Build history of the part. All positions in model axes, mm. Face numbers are marked on the shaded views. A direction names the side the tool comes from. Round coordinates to 2 decimals unless told otherwise and drop trailing zeros. Write each loop counter-clockwise with the first axis right and the second up, starting at its lowest first coordinate (ties: lowest second). Pieces come first, ordered by that corner, then holes. Notation, with made-up numbers: (-16.5, 31) -> (4.5, 31) arc R21 cw to (4.5, 37) -> close; hole circle Ø3 at (39.25, -28.75). An arc over 180 degrees is marked (long way). Answer as CSV lines item,"result".
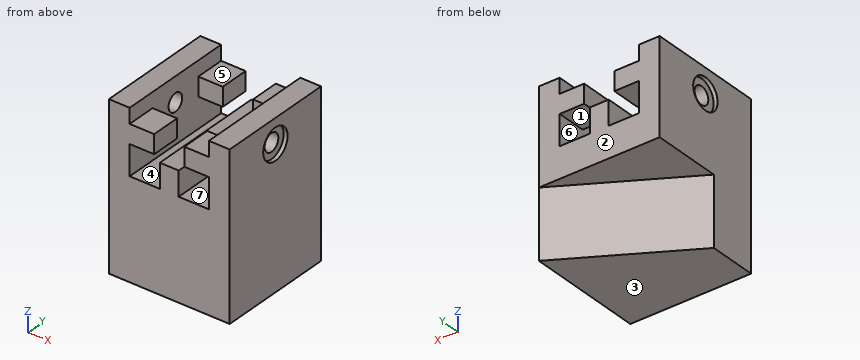
from build123d import *

# Parameters (mm, degrees)
BOSS_EXTRU_1_DEPTH                                = 15
ESQUISSE2_W                                       = 30.8
ESQUISSE2_H                                       = 30
BOSS_EXTRU_2_DEPTH                                = 20
ENL_V_MAT_EXTRU_2_DEPTH                           = 47.870913155
ENL_V_MAT_EXTRU_2_DEPTH_BACK                      = 17.5
ESQUISSE4_W                                       = 4.8
ESQUISSE4_H                                       = 15
ENL_V_MAT_EXTRU_3_DEPTH                           = 6.25
ESQUISSE5_W                                       = 4.8
ESQUISSE5_H                                       = 15
ENL_V_MAT_EXTRU_4_DEPTH                           = 6.25
CHAMBRAGE_POUR_VIS_SIX_PANS_CREUX_M41_D           = 4.5
CHAMBRAGE_POUR_VIS_SIX_PANS_CREUX_M41_DEPTH       = 5.3
CHAMBRAGE_POUR_VIS_SIX_PANS_CREUX_M41_CBORE_D     = 8
CHAMBRAGE_POUR_VIS_SIX_PANS_CREUX_M41_CBORE_DEPTH = 1
CHAMBRAGE_POUR_VIS_SIX_PANS_CREUX_M43_D           = 4.5
CHAMBRAGE_POUR_VIS_SIX_PANS_CREUX_M43_CBORE_D     = 8
CHAMBRAGE_POUR_VIS_SIX_PANS_CREUX_M43_CBORE_DEPTH = 1


with BuildPart() as part:
    # Base → Boss.-Extru.1 (new, symmetric)
    with BuildSketch(Plane(origin=(0, 0, 0), x_dir=(1, 0, 0), z_dir=(0, 1, 0))):
        Polygon((-3.85, -2.4), (-3.85, 2.4), (-10.1, 2.4), (-10.1, 10.1), (-2.4, 10.1), (-2.4, 3.85), (2.4, 3.85), (2.4, 10.1), (10.1, 10.1), (10.1, 2.4), (3.85, 2.4), (3.85, -2.4), (10.1, -2.4), (10.1, -6.25), (15.4, -6.25), (15.4, 15.4), (-15.4, 15.4), (-15.4, -6.25), (-10.1, -6.25), (-10.1, -2.4), align=None)
    extrude(amount=BOSS_EXTRU_1_DEPTH, both=True)

    # Esquisse2 → Boss.-Extru.2 (add)
    with BuildSketch(Plane(origin=(0, 0, -15.4), x_dir=(-1, 0, 0), z_dir=(0, 0, -1))):
        Rectangle(ESQUISSE2_W, ESQUISSE2_H)
    extrude(amount=BOSS_EXTRU_2_DEPTH)

    # Esquisse3 → Enlèv. mat.-Extru.2 (cut, two sides: drawn at the far end of the back side and taken through both)
    with BuildSketch(Plane(origin=(0, 0, -35.4), x_dir=(-1, 0, 0), z_dir=(0, 0, -1)).offset(-ENL_V_MAT_EXTRU_2_DEPTH_BACK)):
        Polygon((-98.531187965, 62.99581375), (-15.4, 15), (15.4, -2.782388291), (98.531187965, -50.778202041), (194.522815465, 115.484173889), (-2.539560466, 229.25818968), align=None)
    extrude(amount=ENL_V_MAT_EXTRU_2_DEPTH + ENL_V_MAT_EXTRU_2_DEPTH_BACK, mode=Mode.SUBTRACT)

    # Esquisse4 → Enlèv. mat.-Extru.3 (cut)
    with BuildSketch(Plane.ZY.offset(-3.85)):
        Rectangle(ESQUISSE4_W, ESQUISSE4_H)
    extrude(amount=-ENL_V_MAT_EXTRU_3_DEPTH, mode=Mode.SUBTRACT)

    # Esquisse5 → Enlèv. mat.-Extru.4 (cut)
    with BuildSketch(Plane(origin=(-3.85, 0, 0), x_dir=(0, 0, -1), z_dir=(1, 0, 0))):
        Rectangle(ESQUISSE5_W, ESQUISSE5_H)
    extrude(amount=-ENL_V_MAT_EXTRU_4_DEPTH, mode=Mode.SUBTRACT)

    # Chambrage pour vis à six pans creux M41
    with Locations(Plane(origin=(15.4, 0, 0), x_dir=(0, 0, -1), z_dir=(1, 0, 0))):
        with Locations((0, 0)):
            CounterBoreHole(CHAMBRAGE_POUR_VIS_SIX_PANS_CREUX_M41_D / 2, CHAMBRAGE_POUR_VIS_SIX_PANS_CREUX_M41_CBORE_D / 2, CHAMBRAGE_POUR_VIS_SIX_PANS_CREUX_M41_CBORE_DEPTH, depth=CHAMBRAGE_POUR_VIS_SIX_PANS_CREUX_M41_DEPTH)

    # Chambrage pour vis à six pans creux M43 (through all)
    with Locations(Plane.ZY.offset(15.4)):
        with Locations((0, 0)):
            CounterBoreHole(CHAMBRAGE_POUR_VIS_SIX_PANS_CREUX_M43_D / 2, CHAMBRAGE_POUR_VIS_SIX_PANS_CREUX_M43_CBORE_D / 2, CHAMBRAGE_POUR_VIS_SIX_PANS_CREUX_M43_CBORE_DEPTH)


solid = part.part
1. Cut at A-A, the plane z = 0. Count the separate pieces of the cut face and the enclosed holes in it, then the cut area to 3 significant figures.
Results found:
separate pieces,"4"
enclosed holes,"0"
area,"451 mm2"
2. Cut at B-B, the plane y = -11.75. Write the cut outline in (x, z).
Results found:
outline,"(-15.4, -35.4) -> (15.4, -35.4) -> (15.4, 6.25) -> (10.1, 6.25) -> (10.1, 2.4) -> (3.85, 2.4) -> (3.85, -2.4) -> (10.1, -2.4) -> (10.1, -10.1) -> (2.4, -10.1) -> (2.4, -3.85) -> (-2.4, -3.85) -> (-2.4, -10.1) -> (-10.1, -10.1) -> (-10.1, -2.4) -> (-3.85, -2.4) -> (-3.85, 2.4) -> (-10.1, 2.4) -> (-10.1, 6.25) -> (-15.4, 6.25) -> close"
3. Which spindle directions (+Z, -Z, +X, -X, +Y, -Y) get a long thin tool onto all of the face, cutting with end or side? Do the marked faces 5, 6 and 7. Say none if no direction does.
Results found:
face 5,"+Z, +Y, -Y"
face 6,"none"
face 7,"+Y, -Y"
4. Cut at D-D, the plane x = 13.5. Write the cut outline in (y, z), then the cut area to 3 significant figures.
Results found:
outline,"(-15, -35.4) -> (13.9, -35.4) -> (13.9, -17.9) -> (15, -17.9) -> (15, 6.25) -> (-15, 6.25) -> close; hole circle Ø4.5 at (0, 0)"
area,"1,210 mm2"
5. Mould opens along Z. For the marked faces 1, 2, 3 and 4 say: +Z half, -Z half, draft (parallel to the pull), parting line (faces both ways), or undercut.
Results found:
face 1,"undercut"
face 2,"draft"
face 3,"-Z half"
face 4,"undercut"
6. Drop flat-ended pins along their axis: pin 1 Ø1 at (x, y) = (-3, 7.5) entering from -Z; pin 2 Ø1.9 at (x, y) = (7, -9.5) entering from +Z; pin 3 Ø5 at (y, z) = (0, 0) entering from -X. Give the stop position or say it passes through.
Results found:
pin 1,"stops at z = -17.9"
pin 2,"stops at z = 2.4"
pin 3,"stops at x = -14.4"
7. Probe line 1 along X through (y, z) = (3.25, -7); line 2 along Y through (x, z) = (14, 0); line 3 along Z through (x, y) = (12.85, 0). List the from-to ranges inside material, lowest first.
Results found:
line 1,"x = -15.4 to -10.1, -2.4 to 2.4, 10.1 to 15.4"
line 2,"y = -15 to -2.25, 2.25 to 15"
line 3,"z = -35.4 to -2.25, 2.25 to 6.25"
8. Cut at C-C, the plane x = -5. Write the cut outline in (y, z).
Results found:
outline,"(-15, -35.4) -> (3.22, -35.4) -> (3.22, -17.9) -> (15, -17.9) -> (15, -10.1) -> (-15, -10.1) -> close; (-15, -2.4) -> (-7.5, -2.4) -> (-7.5, 2.4) -> (-15, 2.4) -> close; (7.5, -2.4) -> (15, -2.4) -> (15, 2.4) -> (7.5, 2.4) -> close"
